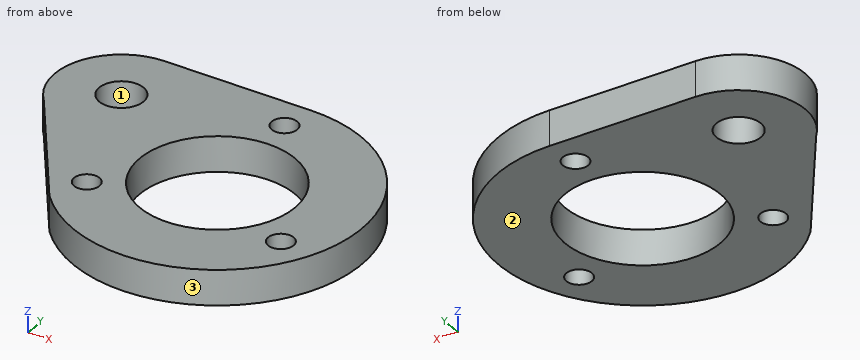
from build123d import *

# Parameters (mm, degrees)
SKETCH1_R           = 3.5
SKETCH1_R_2         = 0.575
SKETCH1_R_3         = 1
BOSS_EXTRUDE1_DEPTH = 1.59


with BuildPart() as part:
    # Sketch1 → Boss-Extrude1 (new body)
    with BuildSketch(Plane.XY):
        with BuildLine():
            Line((38.934590504, 57.571868893), (45.629621497, 57.288743472))
            ThreePointArc((45.629621497, 57.288743472), (51.171586425, 47.893307318), (40.332417108, 46.668560697))
            Line((40.332417108, 46.668560697), (36.48972694, 52.670246074))
            ThreePointArc((36.48972694, 52.670246074), (36.123253783, 55.913581906), (38.934590504, 57.571868893))
        make_face()
        with Locations((45.35498918, 50.794547826)):
            Circle(SKETCH1_R, mode=Mode.SUBTRACT)
        with Locations((45.35498918, 55.794547826)):
            Circle(SKETCH1_R_2, mode=Mode.SUBTRACT)
        with Locations((49.685116199, 48.294547826)):
            Circle(SKETCH1_R_2, mode=Mode.SUBTRACT)
        with Locations((41.024862161, 48.294547826)):
            Circle(SKETCH1_R_2, mode=Mode.SUBTRACT)
        with Locations((38.807837127, 54.574547826)):
            Circle(SKETCH1_R_3, mode=Mode.SUBTRACT)
    extrude(amount=BOSS_EXTRUDE1_DEPTH)


solid = part.part
Check sheet for the modelled part. Datum: model origin and axes. Units: mm. Face numbers are marked on the shaded views. Coordinates: 2 decimals unless noted, no trailing zeros. Write each loop counter-clockwise with the first axis right and the second up, starting at its lowest first coordinate (ties: lowest second). Pieces come first, ordered by that corner, then holes. Notation, with made-up numbers: M -14.5,-20 L 37.5,-20 A24 ccw 37.5,7 Z; hole C 67.25,39 d6. An arc over 180 degrees is marked long. Answer as CSV lines item,"result".
Q1. Cross-section at B-B (y = 50). Record the boundary of the cut face in (x, z), then the cut area to 3 significant figures.
Check result:
outline,"M 38.2,0 L 41.95,0 L 41.95,1.59 L 38.2,1.59 Z; M 48.76,0 L 51.81,0 L 51.81,1.59 L 48.76,1.59 Z"
area,"10.8 mm^2"
Q2. Mould release check, pull along Y, two halves, no side actions. Record for the marked faces 1, 2 and 3: released by +Y, released by -Y, zero draft, split by the parting line, or undercut.
Check result:
face 1,"undercut"
face 2,"zero draft"
face 3,"split by the parting line"
Q3. Material ranges on probe 1 along X at (y, z) = (48.25, 0.55); probe 2 along X at (y, z) = (51.5, 0.7); probe 3 along Y at (x, z) = (47.75, 1.35), recorded low to high. Write a range as from..to.
Check result:
probe 1,"39.32..40.45, 41.6..42.95, 47.76..49.11, 50.26..51.34"
probe 2,"37.24..41.93, 48.78..51.82"
probe 3,"44.75..48.24, 53.35..56.84"
Q4. Cross-section at C-C (z = 0.3). Record the boundary of the cut face in (x, y) (3 decimals).
Check result:
outline,"M 36.49,52.67 L 40.332,46.669 A6.5 ccw long 45.63,57.289 L 38.935,57.572 A3 ccw Z; hole C 38.808,54.575 d2; hole C 41.025,48.295 d1.15; hole C 45.355,50.795 d7; hole C 45.355,55.795 d1.15; hole C 49.685,48.295 d1.15"
Q5. Cross-section at A-A (x = 43.25). Record the boundary of the cut face in (y, z).
Check result:
outline,"M 44.64,0 L 48,0 L 48,1.59 L 44.64,1.59 Z; M 53.59,0 L 57.39,0 L 57.39,1.59 L 53.59,1.59 Z"
Q6. Go/stop test with flat-tipped pins: pin 1 (1.5 mm diameter, centred on x = 42.5, y = 55.5, fed in from -Z); pin 2 (6.5 mm diameter, centred on x = 45.35, y = 50.79, fed in from +Z). Record where each tip stops, or that it passes through.
Check result:
pin 1,"z = 0"
pin 2,"through"
Q7. Cross-section at D-D (y = 46). Record the boundary of the cut face in (x, z), then the cut area to 3 significant figures.
Check result:
outline,"M 40.97,0 L 49.74,0 L 49.74,1.59 L 40.97,1.59 Z"
area,"14.0 mm^2"
